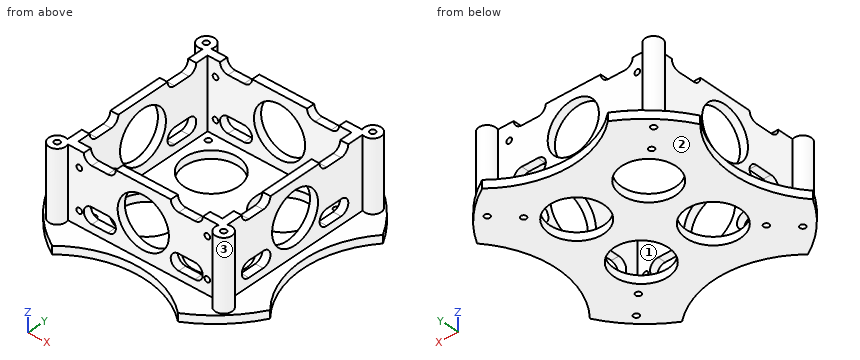
```python
from build123d import *

# Parameters (mm, degrees)
SKETCH_R        = 80
PAD_DEPTH       = 5
PAD001_DEPTH    = 44
SKETCH003_W     = 90
SKETCH003_H     = 90
POCKET_DEPTH    = 44
SKETCH004_R     = 1.75
POCKET001_DEPTH = 49.001
SKETCH005_R     = 17
SKETCH005_R_2   = 60
POCKET002_DEPTH = 5.001
SKETCH006_R     = 16
POCKET003_DEPTH = 119.674913
SKETCH007_R     = 16
POCKET004_DEPTH = 119.674913
SKETCH010_R     = 1.75
POCKET005_DEPTH = 119.674913
SKETCH011_R     = 1.75
POCKET006_DEPTH = 5.001


with BuildPart() as part:
    # Sketch → Pad (new body)
    with BuildSketch(Plane.XY):
        Circle(SKETCH_R)
    extrude(amount=PAD_DEPTH)

    # Sketch002 → Pad001 (new body)
    with BuildSketch(Plane.XY.offset(5)):
        with BuildLine():
            ThreePointArc((-47.145878, 50), (-55.712311, 55.712311), (-50, 47.145878))
            Line((-50, -47.145878), (-50, 47.145878))
            ThreePointArc((-50, -47.145878), (-55.712311, -55.712311), (-47.145878, -50))
            Line((47.145878, -50), (-47.145878, -50))
            ThreePointArc((47.145878, -50), (55.712311, -55.712311), (50, -47.145878))
            Line((50, 47.145878), (50, -47.145878))
            ThreePointArc((50, 47.145878), (55.712311, 55.712311), (47.145878, 50))
            Line((-47.145878, 50), (47.145878, 50))
        make_face()
    extrude(amount=PAD001_DEPTH)

    # Sketch003 → Pocket (cut)
    with BuildSketch(Plane.XY.offset(49)):
        Rectangle(SKETCH003_W, SKETCH003_H)
    extrude(amount=-POCKET_DEPTH, mode=Mode.SUBTRACT)

    # Sketch004 → Pocket001 (cut, through all)
    with BuildSketch(Plane.XY.offset(49)):
        with Locations((-52, -52)):
            Circle(SKETCH004_R)
        with Locations((52, 52)):
            Circle(SKETCH004_R)
        with Locations((52, -52)):
            Circle(SKETCH004_R)
        with Locations((-52, 52)):
            Circle(SKETCH004_R)
    extrude(amount=-POCKET001_DEPTH, mode=Mode.SUBTRACT)

    # Sketch005 → Pocket002 (cut, through all)
    with BuildSketch(Plane.XY.offset(5)):
        with Locations((-22.5, 22.5)):
            Circle(SKETCH005_R)
        with Locations((22.5, 22.5)):
            Circle(SKETCH005_R)
        with Locations((-22.5, -22.5)):
            Circle(SKETCH005_R)
        with Locations((22.5, -22.5)):
            Circle(SKETCH005_R)
        with Locations((0, -115)):
            Circle(SKETCH005_R_2)
        with Locations((-115, 0)):
            Circle(SKETCH005_R_2)
        with Locations((115, 0)):
            Circle(SKETCH005_R_2)
        with Locations((0, 115)):
            Circle(SKETCH005_R_2)
    extrude(amount=-POCKET002_DEPTH, mode=Mode.SUBTRACT)

    # Sketch006 → Pocket003 (cut, through all)
    with BuildSketch(Plane.YZ.offset(50)):
        with Locations((0, 27)):
            Circle(SKETCH006_R)
        with BuildLine():
            ThreePointArc((-32.145847, 20), (-37.145878, 15.000015), (-32.145878, 10))
            Line((-32.145878, 10), (-22.145878, 10))
            ThreePointArc((-22.145878, 10), (-17.145878, 14.999986), (-22.145849, 20))
            Line((-32.145847, 20), (-22.145849, 20))
        make_face()
        with BuildLine():
            ThreePointArc((22.145861, 20), (17.145878, 14.999992), (22.145878, 10))
            Line((22.145878, 10), (32.145878, 10))
            ThreePointArc((32.145878, 10), (37.145878, 15.000009), (32.14586, 20))
            Line((22.145861, 20), (32.14586, 20))
        make_face()
        with BuildLine():
            ThreePointArc((-32.145895, 54), (-37.145878, 49), (-32.145895, 44))
            Line((-32.145895, 44), (-22.145886, 44))
            ThreePointArc((-22.145886, 44), (-17.145878, 48.999999), (-22.145885, 54))
            Line((-32.145895, 54), (-22.145885, 54))
        make_face()
        with BuildLine():
            ThreePointArc((22.145867, 54), (17.145878, 49), (22.145867, 44))
            Line((22.145867, 44), (32.145858, 44))
            ThreePointArc((32.145858, 44), (37.145878, 49), (32.145857, 54))
            Line((22.145867, 54), (32.145857, 54))
        make_face()
    extrude(amount=-POCKET003_DEPTH, mode=Mode.SUBTRACT)

    # Sketch007 → Pocket004 (cut, through all)
    with BuildSketch(Plane.XZ.offset(50)):
        with Locations((0, 27)):
            Circle(SKETCH007_R)
        with BuildLine():
            ThreePointArc((-32.165386, 54), (-37.165371, 48.999992), (-32.165371, 44))
            Line((-32.165371, 44), (-22.165371, 44))
            ThreePointArc((-22.165371, 44), (-17.165371, 49.000008), (-22.165388, 54))
            Line((-32.165386, 54), (-22.165388, 54))
        make_face()
        with BuildLine():
            ThreePointArc((32.189297, 44), (37.189317, 48.99999), (32.189316, 54))
            Line((32.189316, 54), (22.189316, 54))
            ThreePointArc((22.189316, 54), (17.189317, 49.000008), (22.189299, 44))
            Line((32.189297, 44), (22.189299, 44))
        make_face()
        with BuildLine():
            ThreePointArc((-32.145897, 20), (-37.145878, 14.99999), (-32.145878, 10))
            Line((-32.145878, 10), (-22.145878, 10))
            ThreePointArc((-22.145878, 10), (-17.145878, 15.000011), (-22.145899, 20))
            Line((-32.145897, 20), (-22.145899, 20))
        make_face()
        with BuildLine():
            ThreePointArc((22.145901, 20), (17.145878, 15.000011), (22.145878, 10))
            Line((22.145878, 10), (32.145878, 10))
            ThreePointArc((32.145878, 10), (37.145878, 14.999989), (32.1459, 20))
            Line((22.145901, 20), (32.1459, 20))
        make_face()
    extrude(amount=-POCKET004_DEPTH, mode=Mode.SUBTRACT)

    # Sketch010 → Pocket005 (cut, through all)
    with BuildSketch(Plane(origin=(0, 50, 0), x_dir=(-1, 0, 0), z_dir=(0, 1, 0))):
        with Locations((-40, 39)):
            Circle(SKETCH010_R)
        with Locations((-40, 14)):
            Circle(SKETCH010_R)
        with Locations((40, 14)):
            Circle(SKETCH010_R)
        with Locations((40, 39)):
            Circle(SKETCH010_R)
    extrude(amount=-POCKET005_DEPTH, mode=Mode.SUBTRACT)

    # Sketch011 → Pocket006 (cut, through all)
    with BuildSketch(Plane.XY.offset(5)):
        with Locations((39.999999, 40)):
            Circle(SKETCH011_R)
        with Locations((-40.000001, 40)):
            Circle(SKETCH011_R)
        with Locations((-40, -40)):
            Circle(SKETCH011_R)
        with Locations((40, -40)):
            Circle(SKETCH011_R)
    extrude(amount=-POCKET006_DEPTH, mode=Mode.SUBTRACT)


solid = part.part
```
CAD build for the part. Positions are in the model's coordinates, mm. Face numbers are marked on the shaded views. Coordinates: 2 decimals unless noted, no trailing zeros. Loops run counter-clockwise (first coordinate to the right, second up) from the corner with the lowest first, then second, coordinate; pieces in that order, holes last. Notation, with made-up numbers: (87, 30) - (123, 30) arc R21 cw to (123, 59) - close; hole circle Ø2 at (19.25, 61). An arc over 180 degrees is marked (long way). Return JSON: item names as keys, results as strings.
1. Band-saw the part on C-C (y = 25). Give the cut face in (x, z), and give its area (3 significant figures).
Result:
{"outline": "(-60.46, 0) - (-39.32, 0) - (-39.32, 5) - (-45, 5) - (-45, 10) - (-50, 10) - (-50, 5) - (-60.46, 5) - close; (-50, 20) - (-45, 20) - (-45, 44) - (-50, 44) - close; (-5.68, 0) - (5.68, 0) - (5.68, 5) - (-5.68, 5) - close; (39.32, 0) - (60.46, 0) - (60.46, 5) - (50, 5) - (50, 10) - (45, 10) - (45, 5) - (39.32, 5) - close; (45, 20) - (50, 20) - (50, 44) - (45, 44) - close", "area": "558 mm2"}
2. Probe L1, parallel to Y at x = 52, z = 28; L2, parallel to Y at x = 25, z = 32; L3, parallel to Y at x = 40, z = 2.2. List the from-to ranges inside material, lowest first. Write a range as from..to.
Result:
{"L1": "y = -57.25..-53.75, -50.25..-46.75, 46.75..50.25, 53.75..57.25", "L2": "y = -50..-45, 45..50", "L3": "y = -69.28..-41.75, -38.25..38.25, 41.75..69.28"}
3. Band-saw the part on D-D (x = -19.5). Give the cut face in (y, z).
Result:
{"outline": "(-58.26, 0) - (-39.23, 0) - (-39.23, 5) - (-45, 5) - (-45, 10.76) - (-50, 10.76) - (-50, 5) - (-58.26, 5) - close; (-50, 19.24) - (-45, 19.24) - (-45, 44.77) - (-50, 44.77) - close; (-5.77, 0) - (5.77, 0) - (5.77, 5) - (-5.77, 5) - close; (39.23, 0) - (58.26, 0) - (58.26, 5) - (50, 5) - (50, 10.76) - (45, 10.76) - (45, 5) - (39.23, 5) - close; (45, 19.24) - (50, 19.24) - (50, 44.77) - (45, 44.77) - close"}
4. Band-saw the part on A-A (y = 0). Give the cut face in (x, z), and give its area (3 significant figures).
Result:
{"outline": "(-55, 0) - (55, 0) - (55, 5) - (50, 5) - (50, 11) - (45, 11) - (45, 5) - (-45, 5) - (-45, 11) - (-50, 11) - (-50, 5) - (-55, 5) - close; (-50, 43) - (-45, 43) - (-45, 49) - (-50, 49) - close; (45, 43) - (50, 43) - (50, 49) - (45, 49) - close", "area": "670 mm2"}
5. Band-saw the part on B-B (z = 30.5). State how many separate pieces and enclosed holes the cut face has, and give its area (3 significant figures).
Result:
{"separate pieces": "4", "enclosed holes": "4", "area": "1,560 mm2"}
6. Drop flat-ended pins along their axis: pin 1 (4 mm diameter, centred on x = -18.5, z = 31, fed in from +Y); pin 2 (1 mm diameter, centred on x = -4.5, y = -32, fed in from -Z); pin 3 (5 mm diameter, centred on y = -20, z = 22, fed in from +X); pin 4 (2.5 mm diameter, centred on x = 46.5, y = 25, fed in from +Z). Give the stop position or say it passes through.
Result:
{"pin 1": "stops at y = 50", "pin 2": "stops at z = 0", "pin 3": "stops at x = 50", "pin 4": "stops at z = 44"}
7. Mould opens along Y. For the marked faces 1, 2 and 3 say: released by +Y, released by -Y, zero draft, split by the parting line, or undercut.
Result:
{"face 1": "undercut", "face 2": "zero draft", "face 3": "undercut"}
